Here's how the part is built. I have some questions about the finished solid (model axes, mm). A direction names the side the tool comes from. Round coordinates to 2 decimals unless told otherwise and drop trailing zeros. Write each loop counter-clockwise with the first axis right and the second up, starting at its lowest first coordinate (ties: lowest second). Pieces come first, ordered by that corner, then holes. Notation, with made-up numbers: (85, -37) - (106, -37) arc R36 cw to (106, 0) - close; hole circle Ø8 at (-24.5, -8.5). An arc over 180 degrees is marked (long way). Write item = value, one per line. Start each with the question number.
Item 1: If we section it at D-D (x = 43): Please give me the cut outline in (y, z).
Item 2: If we section it at C-C (z = 6.25): Give the number of separate pieces and of enclosed holes in the cut face, and give its area (3 significant figures).
Item 3: If we section it at A-A (y = 0): Please give me the cut outline in (x, z), and give its area (3 significant figures).
Item 4: If we section it at B-B (z = 10.75): Please give me the cut outline in (x, y).
Item 5: For P1, Ø1, axis at x = 13.5, y = 3, coming from the +Z side, with a flat end and sliding along its axis, tell me the tip position at first contact or that it passes through.
Item 6: If I drill on line 1 along Y through (x, z) = (53.2, 6.5); line 2 along Z through (x, y) = (36.5, 2.5); line 3 along Z through (x, y) = (-44, 3.25), over which ranges is the centre line in solid material (lowest first)? Write a range as [from, to].
Item 7: Which directions (+Z, -Z, +X, -X, +Y, -Y) give clear straight access to the entire face, cutting with the end or side of a thin tool? Please do faces 5 (the face through (53.521, 0.064, 7.947)), 6 (the face through (12, 0, 3)), 7 (the face through (4, -6.5, 2)).
Item 8: Thinking about a two-plate mould opening in X: for faces 1 (the face through (52, 0, 9)), 2 (the face through (-40.93, -2.98, 4.7)), 3 (the face through (14, 0, 0)), 4 (the face through (55, -2, 6)), which applies, pulls with the +X half, pulls with the -X half, needs draft (parallel to the pull), parting line crosses it, or undercut?
```python
from build123d import *

# Parameters (mm, degrees)
SKETCH1_W           = 110
SKETCH1_H           = 13
BOSS_EXTRUDE1_DEPTH = 50
CUT_EXTRUDE1_DEPTH  = 76.45859792
CUT_EXTRUDE2_DEPTH  = 76.45859792
SKETCH4_R           = 2
CUT_EXTRUDE3_DEPTH  = 62.317648321
SKETCH5_W           = 3
SKETCH5_H           = 13
BOSS_EXTRUDE2_DEPTH = 10
SKETCH6_R           = 1.448838416
CUT_EXTRUDE5_DEPTH  = 12


with BuildPart() as part:
    # Sketch1 → Boss-Extrude1 (new body)
    with BuildSketch(Plane.XY):
        Rectangle(SKETCH1_W, SKETCH1_H)
    extrude(amount=BOSS_EXTRUDE1_DEPTH)

    # Sketch2 → Cut-Extrude1 (cut, through all)
    with BuildSketch(Plane.XZ.offset(6.5)):
        Polygon((-55, 9.270509831), (-26.468304511, 0), (-55, 0), align=None)
    extrude(amount=-CUT_EXTRUDE1_DEPTH, mode=Mode.SUBTRACT)

    # Sketch3 → Cut-Extrude2 (cut, through all)
    with BuildSketch(Plane.XZ.offset(6.5)):
        Polygon((-55, 12.424896504), (-25.99315119, 3), (55, 3), (55, 50), (-55, 50), align=None)
    extrude(amount=-CUT_EXTRUDE2_DEPTH, mode=Mode.SUBTRACT)

    # Sketch4 → Cut-Extrude3 (cut, through all)
    with BuildSketch(Plane(origin=(-2.527498175, 0, -7.778839522), x_dir=(-0.9510565162951533, 0, 0.30901699437494845), z_dir=(-0.30901699437494845, 0, -0.9510565162951533))):
        with Locations((40.172853481, 0)):
            Circle(SKETCH4_R)
    extrude(amount=-CUT_EXTRUDE3_DEPTH, mode=Mode.SUBTRACT)

    # Sketch5 → Boss-Extrude2 (add)
    with BuildSketch(Plane.XY.offset(3)):
        with Locations((53.5, 0)):
            Rectangle(SKETCH5_W, SKETCH5_H)
    extrude(amount=BOSS_EXTRUDE2_DEPTH)

    # Sketch6 → Cut-Extrude5 (cut)
    with BuildSketch(Plane(origin=(55, 0, 0), x_dir=(0, 0, -1), z_dir=(1, 0, 0))):
        with Locations((-6.5, 0)):
            Circle(SKETCH6_R)
    extrude(amount=-CUT_EXTRUDE5_DEPTH, mode=Mode.SUBTRACT)


solid = part.part
```
Reply:
q1.outline = (-6.5, 0) - (6.5, 0) - (6.5, 3) - (-6.5, 3) - close
q2.separate_pieces = 3
q2.enclosed_holes = 1
q2.area = 143 mm2
q3.outline = (-55, 9.27) - (-42.64, 5.25) - (-41.71, 8.11) - (-55, 12.42) - close; (-38.83, 4.02) - (-26.47, 0) - (55, 0) - (55, 5.05) - (52, 5.05) - (52, 3) - (-25.99, 3) - (-37.9, 6.87) - close; (52, 7.95) - (55, 7.95) - (55, 13) - (52, 13) - close
q3.area = 344 mm2
q4.outline = (-55, -6.5) - (-49.85, -6.5) - (-49.85, 6.5) - (-55, 6.5) - close; (52, -6.5) - (55, -6.5) - (55, 6.5) - (52, 6.5) - close
q5.P1 = 3
q6.line_1 = [-6.5, -1.45], [1.45, 6.5]
q6.line_2 = [0, 3]
q6.line_3 = [5.7, 8.85]
q7.face_5 = +X
q7.face_6 = +Z, +Y, -Y
q7.face_7 = +Z, -Z, +X, -X, -Y
q8.face_1 = undercut
q8.face_2 = pulls with the -X half
q8.face_3 = needs draft
q8.face_4 = pulls with the +X half
